Read the model definition and answer for the solid it produces. Units are mm, in the model's axes. Coordinates: 2 decimals unless noted, no trailing zeros. Order: outer loops, then holes, each group sorted by start corner. A loop starts at its lowest first (then second) coordinate and runs counter-clockwise, first axis right, second up. Notation, with made-up numbers: (68.5, 55.5) - (83.5, 55.5) arc R16 cw to (83.5, 74.5) - close; hole circle Ø5 at (78.5, 53.5). An arc over 180 degrees is marked (long way). Use one line per item in the form item = value.
```python
from build123d import *

# Parameters (mm, degrees)
F0_R          = 0.75
F1_DEPTH      = 14.986
F3_DEPTH      = 114.3
F5_DEPTH      = 25.4
F5_DEPTH_BACK = 25.4


# Not quite as in the source:
# - a feature names something its author has since deleted; it is built from what else it names


with BuildPart() as f1:
    # F0 (on Top) → F1 (new body)
    with BuildSketch(Plane.XY):
        Polygon((59.3341242821, 21.43125), (-59.3341242821, 19.05), (-59.3341242821, -19.05), (59.3341242821, -21.43125), align=None)
        with Locations((-49.3341242821, -14.2496579055)):
            Circle(F0_R, mode=Mode.SUBTRACT)
        with Locations((-49.3341242821, -4.2496579055)):
            Circle(F0_R, mode=Mode.SUBTRACT)
        with Locations((-49.3341242821, 4.2496579055)):
            Circle(F0_R, mode=Mode.SUBTRACT)
        with Locations((-49.3341242821, 14.2496579055)):
            Circle(F0_R, mode=Mode.SUBTRACT)
    extrude(amount=F1_DEPTH)

    # F2 (on face) → F3 (intersect)
    with BuildSketch(Plane.YZ.offset(59.3341242821)):
        with BuildLine():
            Line((21.43125, 14.986), (-21.43125, 14.986))
            ThreePointArc((-21.43125, 14.986), (-13.0755370179, 4.1181258353), (-1.54e-08, 0))
            ThreePointArc((-1.54e-08, 0), (13.0755370052, 4.1181258265), (21.43125, 14.986))
        make_face()
    extrude(amount=-F3_DEPTH, mode=Mode.INTERSECT)

    # F4 (on Front) → F5 (cut, two sides)
    with BuildSketch(Plane.XZ) as f5_sk:
        Polygon((-54.9658757179, 14.986), (-54.9658757179, 10.3923923096), (59.3341242821, 14.986), align=None)
    extrude(amount=-F5_DEPTH, mode=Mode.SUBTRACT)
    extrude(f5_sk.sketch, amount=F5_DEPTH_BACK, mode=Mode.SUBTRACT)


solid = f1.part
```
(1) Section C-C, the plane y = -8.5 is taken. Write down the section's boundary in (x, z).
Answer list:
outline = (-54.97, 1.64) - (59.33, 1.64) - (59.33, 14.99) - (-54.97, 10.39) - close
(2) Section D-D, the plane x = 31.5 is taken. Write down the section's boundary in (y, z), then the cut area to 3 significant figures.
Answer list:
outline = (-20.87, 13.6) arc R22.82 ccw to (20.87, 13.6) - (20.87, 13.87) - (-20.87, 13.87) - close
area = 420 mm2
(3) Straight lines are drawn through the part: L1, parallel to Z at x = 27, y = 17; L2, parallel to Y at x = 20.5, z = 8.5; L3, parallel to Z at x = 46, y = 2. For each, find the intervals that lie inside material, in ascending order.
Answer list:
L1 = 7.6 to 13.69
L2 = -17.77 to 17.77
L3 = 0.09 to 14.45
(4) Given pin 1 Ø2 at (x, y) = (-49.33, -4.25) entering from +Z; pin 2 Ø1.2 at (x, y) = (-49.33, 14.25) entering from +Z; pin 3 Ø3 at (x, y) = (-6.5, -4) entering from -Z; pin 4 Ø6 at (x, y) = (3.5, 14.5) entering from +Z, each flat-ended and moving along its own axis, determine where each tip first touches the part or whether it passes through.
Answer list:
pin_1 = 10.66
pin_2 = through
pin_3 = 0.14
pin_4 = 12.86
(5) Section A-A, the plane z = 6 is taken. Write down the section's boundary in (x, y).
Answer list:
outline = (-54.97, -15.42) - (59.33, -15.42) - (59.33, 15.42) - (-54.97, 15.42) - close; hole circle Ø1.5 at (-49.33, -14.25); hole circle Ø1.5 at (-49.33, -4.25); hole circle Ø1.5 at (-49.33, 4.25); hole circle Ø1.5 at (-49.33, 14.25)
(6) Section B-B, the plane x = -23.5 is taken. Write down the section's boundary in (y, z).
Answer list:
outline = (-19.77, 11.42) arc R22.82 ccw to (19.77, 11.42) - (19.77, 11.66) - (-19.77, 11.66) - close
